from build123d import *

# Parameters (mm, degrees)
F1_DEPTH = 2
F3_DEPTH = 3
F5_DEPTH = 1
F6_R     = 1


with BuildPart() as f1:
    # F0 (on Top) → F1 (new body)
    with BuildSketch(Plane.XY):
        with BuildLine():
            Line((55.00297, 100.110456), (-44.382804, 100.110456))
            ThreePointArc((-44.382804, 100.110456), (-51.276236, 97.354806), (-54.37049, 90.606577))
            Line((-54.37049, 90.606577), (-55.390746, 70.067208))
            ThreePointArc((-55.390746, 70.067208), (-52.64741, 62.677656), (-45.40306, 59.571087))
            Line((-45.40306, 59.571087), (-25.153022, 59.571087))
            ThreePointArc((-25.153022, 59.571087), (-18.081955, 56.642155), (-15.153022, 49.571087))
            Line((-15.153022, 49.571087), (-15.153022, -19.336576))
            ThreePointArc((-15.153022, -19.336576), (-17.669577, -25.969679), (-23.952632, -29.264268))
            Line((-23.952632, -29.264268), (-40.499641, -31.265022))
            ThreePointArc((-40.499641, -31.265022), (-46.782696, -34.559611), (-49.299251, -41.192713))
            Line((-49.299251, -41.192713), (-49.299251, -54.753145))
            ThreePointArc((-49.299251, -54.753145), (-46.370319, -61.824213), (-39.299251, -64.753145))
            Line((-39.299251, -64.753145), (39.760375, -64.753145))
            ThreePointArc((39.760375, -64.753145), (46.831443, -61.824213), (49.760375, -54.753145))
            Line((49.760375, -54.753145), (49.760375, -40.710986))
            ThreePointArc((49.760375, -40.710986), (47.424223, -34.287168), (41.507289, -30.864753))
            Line((41.507289, -30.864753), (34.742437, -29.664537))
            ThreePointArc((34.742437, -29.664537), (28.825503, -26.242122), (26.489351, -19.818304))
            Line((26.489351, -19.818304), (26.489351, 54.364799))
            ThreePointArc((26.489351, 54.364799), (27.48312, 58.710809), (30.26691, 62.193032))
            Line((30.26691, 62.193032), (30.519926, 62.394148))
            ThreePointArc((30.519926, 62.394148), (32.537261, 63.638791), (34.790872, 64.37365))
            Line((34.790872, 64.37365), (56.954466, 68.783654))
            ThreePointArc((56.954466, 68.783654), (62.733266, 72.247689), (65.00297, 78.591389))
            Line((65.00297, 78.591389), (65.00297, 90.110456))
            ThreePointArc((65.00297, 90.110456), (62.074038, 97.181524), (55.00297, 100.110456))
        make_face()
    extrude(amount=F1_DEPTH)

    # F2 (on face) → F3 (join)
    with BuildSketch(Plane.XY.offset(2)):
        with BuildLine():
            ThreePointArc((5, 95.998436), (1.464466, 94.53397), (0, 90.998436))
            Line((0, 90.998436), (0, -52.06298))
            ThreePointArc((0, -52.06298), (1.464466, -55.598514), (5, -57.06298))
            Line((5, -57.06298), (9.289023, -57.06298))
            ThreePointArc((9.289023, -57.06298), (12.824557, -55.598514), (14.289023, -52.06298))
            Line((14.289023, -52.06298), (14.289023, 90.998436))
            ThreePointArc((14.289023, 90.998436), (12.824557, 94.53397), (9.289023, 95.998436))
            Line((9.289023, 95.998436), (5, 95.998436))
        make_face()
    extrude(amount=F3_DEPTH)

    # F4 (on face) → F5 (join)
    with BuildSketch(Plane.XY.offset(2)):
        with BuildLine():
            Line((-39.299251, -64.753145), (-40.499641, -31.265022))
            ThreePointArc((-40.499641, -31.265022), (-46.782696, -34.559611), (-49.299251, -41.192713))
            Line((-49.299251, -41.192713), (-49.299251, -54.753145))
            ThreePointArc((-49.299251, -54.753145), (-46.370319, -61.824213), (-39.299251, -64.753145))
        make_face()
        with BuildLine():
            Line((41.507289, -30.864753), (39.760375, -64.753145))
            ThreePointArc((39.760375, -64.753145), (46.831443, -61.824213), (49.760375, -54.753145))
            Line((49.760375, -54.753145), (49.760375, -40.710986))
            ThreePointArc((49.760375, -40.710986), (47.424223, -34.287168), (41.507289, -30.864753))
        make_face()
        with BuildLine():
            Line((-45.40306, 59.571087), (-44.382804, 100.110456))
            ThreePointArc((-44.382804, 100.110456), (-51.276236, 97.354806), (-54.37049, 90.606577))
            Line((-54.37049, 90.606577), (-55.390746, 70.067208))
            ThreePointArc((-55.390746, 70.067208), (-52.64741, 62.677656), (-45.40306, 59.571087))
        make_face()
        with BuildLine():
            ThreePointArc((65.00297, 90.110456), (62.074038, 97.181524), (55.00297, 100.110456))
            Line((55.00297, 100.110456), (56.954466, 68.783654))
            ThreePointArc((56.954466, 68.783654), (62.733266, 72.247689), (65.00297, 78.591389))
            Line((65.00297, 78.591389), (65.00297, 90.110456))
        make_face()
    extrude(amount=F5_DEPTH)

    # F6
    f6_edges = [f1.edges().sort_by_distance(p)[0] for p in [
        (46.831443, -61.824213, 3),
        (49.760375, -47.732065, 3),
        (47.424223, -34.287168, 3),
        (-49.299251, -47.972929, 3),
        (-46.782696, -34.559611, 3),
        (-54.880618, 80.336892, 3),
        (65.00297, 84.350923, 3),
    ]]
    fillet(f6_edges, radius=F6_R)


solid = f1.part
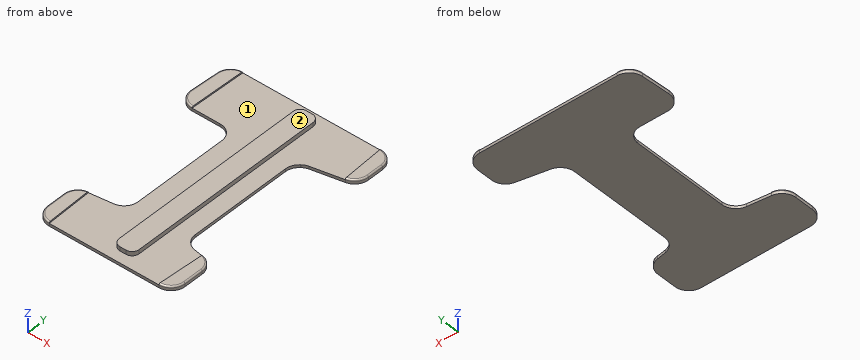
Check sheet for the modelled part. Datum: model origin and axes. Units: mm. Face numbers are marked on the shaded views. Round coordinates to 2 decimals unless told otherwise and drop trailing zeros. Order: outer loops, then holes, each group sorted by start corner. A loop starts at its lowest first (then second) coordinate and runs counter-clockwise, first axis right, second up.
(1) Draft check along X on the marked faces 1 and 2. Enter one of: pulls with the +X half, pulls with the -X half, needs draft (parallel to the pull), parting line crosses it, or undercut.
(2) Cross-section at B-B, the plane z = 1.1. Enter the section's corners in (x, y), and give its area (3 significant figures).
(3) Cross-section at A-A, the plane x = -37.5. Enter the section's corners in (y, z), and give its area (3 significant figures).
(4) Go/stop test with flat-tipped pins: P1, Ø2, axis at y = 18.5, z = 1.5, coming from the +X side; P2, Ø1.6, axis at y = 13, z = 1, coming from the -X side; P3, Ø4.5, axis at x = -41.5, y = -42, coming from the +Z side. Record where each tip stops, or that it passes through.
(5) Scan lines: probe 1 along X at (y, z) = (71, 2.7); probe 2 along X at (y, z) = (-24.5, 4.55); probe 3 along X at (y, z) = (25.5, 1.6). Record each from-to range of solid material in increasing order.
(6) Cross-section at C-C, the plane x = 11. Enter the section's corners in (y, z).
Check sheet entries:
1. face 1: undercut
1. face 2: needs draft
2. outline: (-55.39, 70.07) arc R10 ccw to (-45.4, 59.57) - (-25.15, 59.57) arc R10 cw to (-15.15, 49.57) - (-15.15, -19.34) arc R10 cw to (-23.95, -29.26) - (-40.5, -31.27) arc R10 ccw to (-49.3, -41.19) - (-49.3, -54.75) arc R10 ccw to (-39.3, -64.75) - (39.76, -64.75) arc R10 ccw to (49.76, -54.75) - (49.76, -40.71) arc R10 ccw to (41.51, -30.86) - (34.74, -29.66) arc R10 cw to (26.49, -19.82) - (26.49, 54.36) arc R10 cw to (30.27, 62.19) - (30.52, 62.39) arc R10 cw to (34.79, 64.37) - (56.95, 68.78) arc R10 ccw to (65, 78.59) - (65, 90.11) arc R10 ccw to (55, 100.11) - (-44.38, 100.11) arc R10 ccw to (-54.37, 90.61) - close
2. area: 11,700 mm2
3. outline: (-64.75, 0) - (-30.9, 0) - (-30.9, 2) - (-64.75, 2) - close; (59.57, 0) - (100.11, 0) - (100.11, 2) - (59.57, 2) - close
3. area: 149 mm2
4. P1: stops at x = 26.49
4. P2: stops at x = -15.15
4. P3: stops at z = 3
5. probe 1: x = -55.06 to -45.12, 0 to 14.29, 56.82 to 61.06
5. probe 2: x = 0 to 14.29
5. probe 3: x = -15.15 to 26.49
6. outline: (-64.75, 0) - (100.11, 0) - (100.11, 2) - (95.7, 2) - (95.7, 5) - (-56.76, 5) - (-56.76, 2) - (-64.75, 2) - close
